from build123d import *

# Parameters (mm, degrees)
SKETCH_1_W               = 23
SKETCH_1_H               = 23
SKETCH_1_W_2             = 13
SKETCH_1_H_2             = 13
EXTRUDE_1_DEPTH          = 35
SKETCH_2_R               = 1.65
CUT_EXTRUDE_1_DEPTH      = 34
SKETCH_4_W               = 23
SKETCH_4_H               = 23
SKETCH_4_R               = 3
EXTRUDE_2_DEPTH          = 3.5
SKETCH_5_W               = 23
SKETCH_5_H               = 23
SKETCH_5_W_2             = 13
SKETCH_5_H_2             = 13
EXTRUDE_1_2_DEPTH        = 54
SKETCH_6_R               = 1.65
CUT_EXTRUDE_2_DEPTH      = 39
SKETCH_7_W               = 13
SKETCH_7_H               = 13
CUT_EXTRUDE_3_DEPTH      = 13
CHAMFER_1_SIZE           = 3
SKETCH_8_W               = 80.5
SKETCH_8_H               = 35
CUT_EXTRUDE_4_DEPTH      = 11.5
EXTRUDE_3_DEPTH          = 6.5
FILLET_1_R               = 10
FILLET_2_R               = 10
SKETCH_10_R              = 1.65
CUT_EXTRUDE_5_DEPTH      = 28.5
CHAMFER_4_SIZE           = 3
CHAMFER_START            = 6.5
CHAMFER_5_DEPTH          = 11.5
CUT_EXTRUDE_6_DEPTH      = 106
CUT_EXTRUDE_6_DEPTH_BACK = 86
SKETCH_12_W              = 100.531840745
SKETCH_12_H              = 30.474622789
SKETCH_13_W              = 10
SKETCH_13_H              = 23
EXTRUDE_5_DEPTH          = 10
CHAMFER_13_SIZE          = 10
CHAMFER_14_SIZE          = 10
CHAMFER_15_SIZE          = 5
CHAMFER_16_SIZE          = 5
CHAMFER_17_SIZE          = 1.5


with BuildPart() as part:
    # 草图1 → Extrude 1 (new body)
    with BuildSketch(Plane.XY):
        with Locations((6.5, 6.5)):
            Rectangle(SKETCH_1_W, SKETCH_1_H)
        with Locations((6.5, 6.5)):
            Rectangle(SKETCH_1_W_2, SKETCH_1_H_2, mode=Mode.SUBTRACT)
    extrude(amount=EXTRUDE_1_DEPTH)

    # 草图2 → 切除-拉伸1 (cut)
    with BuildSketch(Plane.XZ.offset(5)):
        with Locations(Location((6.5, 25, 0), (0, 0, 270))):
            Circle(SKETCH_2_R)
    extrude(amount=-CUT_EXTRUDE_1_DEPTH, mode=Mode.SUBTRACT)

    # 草图4 → 凸台-拉伸2 (add)
    with BuildSketch(Plane(origin=(18, 0, 0), x_dir=(0, 0, -1), z_dir=(1, 0, 0))):
        with Locations((-11.5, 6.5)):
            Rectangle(SKETCH_4_W, SKETCH_4_H)
        with Locations(Location((-11.5, 6.5, 0), (0, 0, 90))):
            Circle(SKETCH_4_R, mode=Mode.SUBTRACT)
    extrude(amount=EXTRUDE_2_DEPTH)

    # 草图5 → Extrude 1 2 (add)
    with BuildSketch(Plane(origin=(21.5, 0, 0), x_dir=(0, 0, -1), z_dir=(1, 0, 0))):
        with Locations((-11.5, 6.5)):
            Rectangle(SKETCH_5_W, SKETCH_5_H)
        with Locations((-11.5, 6.5)):
            Rectangle(SKETCH_5_W_2, SKETCH_5_H_2, mode=Mode.SUBTRACT)
    extrude(amount=EXTRUDE_1_2_DEPTH)

    # 草图6 → 切除-拉伸2 (cut)
    with BuildSketch(Plane(origin=(0, 18, 0), x_dir=(1, 0, 0), z_dir=(0, 1, 0))):
        with Locations(Location((65.5, -11.5, 0), (0, 0, 270))):
            Circle(SKETCH_6_R)
    extrude(amount=-CUT_EXTRUDE_2_DEPTH, mode=Mode.SUBTRACT)

    # 草图7 → 切除-拉伸3 (cut)
    with BuildSketch(Plane(origin=(21.5, 0, 0), x_dir=(0, 0, -1), z_dir=(1, 0, 0))):
        with Locations((-11.5, 6.5)):
            Rectangle(SKETCH_7_W, SKETCH_7_H)
    extrude(amount=-CUT_EXTRUDE_3_DEPTH, mode=Mode.SUBTRACT)

    # 倒角1
    chamfer_1_edges = [part.edges().sort_by_distance(p)[0] for p in [
        (13, 6.5, 18),
    ]]
    chamfer(chamfer_1_edges, length=CHAMFER_1_SIZE)

    # 草图8 → 切除-拉伸4 (cut)
    with BuildSketch(Plane.XZ.offset(5)):
        with Locations((35.25, 17.5)):
            Rectangle(SKETCH_8_W, SKETCH_8_H)
    extrude(amount=-CUT_EXTRUDE_4_DEPTH, mode=Mode.SUBTRACT)

    # 草图9 → 凸台-拉伸3 (add)
    with BuildSketch(Plane.XZ.offset(-13)):
        Polygon((13, 5), (0, 16), (0, 0), (13, 0), align=None)
    extrude(amount=EXTRUDE_3_DEPTH)

    # 圆角1
    fillet_1_edges = [part.edges().sort_by_distance(p)[0] for p in [
        (-5, 12.25, 0),
    ]]
    fillet(fillet_1_edges, radius=FILLET_1_R)

    # 圆角2
    fillet_2_edges = [part.edges().sort_by_distance(p)[0] for p in [
        (18, 12.25, 23),
    ]]
    fillet(fillet_2_edges, radius=FILLET_2_R)

    # 草图10 → 切除-拉伸5 (cut)
    with BuildSketch(Plane.XZ.offset(-6.5)):
        with Locations(Location((2, 7, 0), (0, 0, 270))):
            Circle(SKETCH_10_R)
        with Locations(Location((18, 23, 0), (0, 0, 270))):
            Circle(SKETCH_10_R)
    extrude(amount=-CUT_EXTRUDE_5_DEPTH, mode=Mode.SUBTRACT)

    # 倒角4
    chamfer_4_edges = [part.edges().sort_by_distance(p)[0] for p in [
        (75.5, 18, 11.5),
        (6.5, 18, 35),
    ]]
    chamfer(chamfer_4_edges, length=CHAMFER_4_SIZE)

    # 倒角5: read off the stored shape, not the designer's step
    # 倒角5 outline → 倒角5 (cut)
    with BuildSketch(Plane(origin=(0, 0, 0), x_dir=(1, 0, 0), z_dir=(0, 1, 0)).offset(CHAMFER_START)):
        Polygon((72.5, 0), (75.5, -3), (75.5, 0), align=None)
        Polygon((-5, -35), (-2, -35), (-5, -32), align=None)
        with BuildLine():
            ThreePointArc((18, -33), (18.007410169, -32.615099398), (18.029629695, -32.230769231))
            Line((18.029629695, -32.230769231), (15.038518603, -35))
            Line((15.038518603, -35), (18, -35))
            Line((18, -35), (18, -33))
        make_face()
        Polygon((75.5, -20), (72.5, -23), (75.5, -23), align=None)
    extrude(amount=CHAMFER_5_DEPTH, mode=Mode.SUBTRACT)


with BuildPart() as body_2:
    # Split Bodies 1: the piece on the far side of the plane
    add(part.part)
    split(bisect_by=Plane.YZ.offset(50.5), keep=Keep.BOTTOM)


with BuildPart() as part_1:
    add(part.part)

    # Split Bodies 1
    split(bisect_by=Plane.YZ.offset(50.5), keep=Keep.TOP)


with BuildPart() as part_2:
    # Move Body 1: read off the stored shape, not the designer's step
    # Move Body 1: moved
    add(part_1.part.moved(Location((0, 10, 0))))

    # Combine 1: union body 2
    add(body_2.part)


with BuildPart() as body_2_2:
    # 镜向1: mirrored copy
    add(part_2.part.mirror(Plane(origin=(-5, 28, 35), x_dir=(0, 0, 1), z_dir=(0, -1, 0))))

    # 草图13 → 凸台-拉伸5 (add)
    with BuildSketch(Plane.XZ.offset(-38)):
        with Locations((45.5, 11.5)):
            Rectangle(SKETCH_13_W, SKETCH_13_H)
    extrude(amount=EXTRUDE_5_DEPTH)

    # 倒角13
    # the kernel refuses this chamfer: 10 mm, written as the material it takes off along each edge
    with BuildSketch(Plane(origin=(50.5, 43, 5), x_dir=(0, -1, 0), z_dir=(0, 0, 1))) as chamfer_13_piece_1:
        Polygon((CHAMFER_13_SIZE, 0), (0, -CHAMFER_13_SIZE), (0, 0), align=None)
    extrude(amount=13, mode=Mode.SUBTRACT)

    # 倒角14
    chamfer_14_edges = [body_2_2.edges().sort_by_distance(p)[0] for p in [
        (50.5, 49.5, 2.5),
        (50.5, 49.5, 20.5),
    ]]
    chamfer(chamfer_14_edges, length=CHAMFER_14_SIZE - 0.0001)  # a hair under: the kernel refuses the full size

    # 倒角15
    chamfer_15_edges = [body_2_2.edges().sort_by_distance(p)[0] for p in [
        (40.5, 38, 11.5),
    ]]
    chamfer(chamfer_15_edges, length=CHAMFER_15_SIZE)

    # 倒角16
    chamfer_16_edges = [body_2_2.edges().sort_by_distance(p)[0] for p in [
        (40.5, 28, 11.5),
    ]]
    chamfer(chamfer_16_edges, length=CHAMFER_16_SIZE - 0.0001)  # a hair under: the kernel refuses the full size

    # 倒角17
    chamfer_17_edges = [body_2_2.edges().sort_by_distance(p)[0] for p in [
        (40.5, 32.99995, 23),
        (42.99995, 30.49995, 23),
        (38, 35.5, 23),
        (58.99995, 28, 23),
        (31.75, 38, 23),
        (40.5, 32.99995, 0),
        (42.99995, 30.49995, 0),
        (38, 35.5, 0),
        (58.99995, 28, 0),
        (20.25, 38, 0),
        (-2.071067812, 38, 2.928932188),
        (-5, 38, 21),
        (21.291796068, 38, 25.583801513),
    ]]
    chamfer(chamfer_17_edges, length=CHAMFER_17_SIZE)


with BuildPart() as part_3:
    add(part_2.part)

    # 草图12 → 切除-拉伸6 (cut, two sides: drawn at the far end of the back side and taken through both)
    with BuildSketch(Plane.XY.offset(23).offset(-CUT_EXTRUDE_6_DEPTH_BACK)):
        with Locations((32.005641973, 12.762688605)):
            Rectangle(SKETCH_12_W, SKETCH_12_H)
    extrude(amount=CUT_EXTRUDE_6_DEPTH + CUT_EXTRUDE_6_DEPTH_BACK, mode=Mode.SUBTRACT)


solid = body_2_2.part
Design review of the part built by this model. Coordinates are the model's own, in mm. A direction names the side the tool comes from. Coordinates: 2 decimals unless noted, no trailing zeros. Order: outer loops, then holes, each group sorted by start corner. A loop starts at its lowest first (then second) coordinate and runs counter-clockwise, first axis right, second up. Notation, with made-up numbers: (35, 64.25) -> (70, 64.25) arc R32 ccw to (70, 100.25) -> close; hole circle Ø8 at (-24.5, 17.5). An arc over 180 degrees is marked (long way). Use one line per item in the form item = value. Start each with the question number.
(1) The part is to be moulded in two halves that separate along Z. For faces 6 (the flat face through (20.8, 38.8, 0.7)), 7 (the flat face through (44, 41, 5)), 8 (the cylindrical face through (2.07, 43.83, 8.65)), 9 (the flat face through (45, 45, 20)), say which applies: +Z half, -Z half, draft (parallel to the pull), parting line (faces both ways), or undercut.
(2) Add section B-B on x = 65.5. State the section outline as (y, z) points.
(3) Add section D-D on y = 30.25. State the section outline as (x, z) points.
(4) Add section A-A on y = 47.5. State the section outline as (x, z) points.
(5) For probe 1 along Y at (x, z) = (9, 17); probe 2 along X at (y, z) = (40.3, 25); probe 3 along X at (y, z) = (47.25, 19), list the stretches that pass through material, from the lowest coordinate up.
(6) Insertion check: pin 1 (4.5 mm diameter, centred on x = 18, z = 23, fed in from -Y); pin 2 (10.5 mm diameter, centred on x = 67.5, z = 13.5, fed in from +Y); pin 3 (5 mm diameter, centred on x = 35.5, z = 7, fed in from -Y). Each pin has a flat end and moves straight along its axis. Give the tip position at first contact, or say it passes through.
(7) For faces 1 (the conical face through (-1.13, 38.26, 3.74)), 2 (the flat face through (6.591, 46.204, 10.423)), 3 (the flat face through (63, 39.5, 21)), 4 (the flat face through (16, 38, 17)), 5 (the flat face through (32.1, 38.7, 22.2)), list the 3-axis set-ups (+Z, -Z, +X, -X, +Y, -Y) from which the entire face can be reached by the end or side of a thin tool; tool diameter is ignored.
Answer block:
q1.face_6 = -Z half
q1.face_7 = undercut
q1.face_8 = undercut
q1.face_9 = draft
q2.outline = (28, 1.5) -> (29.5, 0) -> (39.5, 0) -> (39.5, 5) -> (33, 5) -> (33, 9.85) -> (28, 9.85) -> close; (28, 13.15) -> (33, 13.15) -> (33, 18) -> (39.5, 18) -> (39.5, 23) -> (29.5, 23) -> (28, 21.5) -> close
q3.outline = (43.25, 1.5) -> (45.37, 0) -> (72.5, 0) -> (74.75, 2.25) -> (74.75, 20.75) -> (72.5, 23) -> (45.37, 23) -> (43.25, 21.5) -> close; hole circle Ø3.3 at (65.5, 11.5)
q4.outline = (-5, 10) arc R10 ccw to (5, 0) -> (42.5, 0) -> (42.5, 5) -> (13, 5) -> (0, 16) -> (0, 35) -> (-2, 35) -> (-5, 32) -> close; (13, 21) -> (16, 18) -> (42.5, 18) -> (42.5, 23) -> (28, 23) arc R10 cw to (18.03, 32.23) -> (15.04, 35) -> (13, 35) -> close; hole circle Ø3.3 at (2, 7); hole circle Ø3.3 at (18, 23)
q5.probe_1 = 38 to 43
q5.probe_2 = -5 to 4.85, 8.15 to 22
q5.probe_3 = -5 to 0, 15 to 42.75
q6.pin_1 = 38
q6.pin_2 = 39.5
q6.pin_3 = 35.5
q7.face_1 = -Z, -X, -Y
q7.face_2 = +Z, +X, +Y
q7.face_3 = +Z, -Z, +X, +Y
q7.face_4 = +Z, -Z, -X, -Y
q7.face_5 = +Z, -Y
